Source: CAD feature listing. Evaluate the final solid. Frame: model axes, mm. Round coordinates to 2 decimals unless told otherwise and drop trailing zeros. Order: outer loops, then holes, each group sorted by start corner. A loop starts at its lowest first (then second) coordinate and runs counter-clockwise, first axis right, second up. Notation, with made-up numbers: (52.25, 40.5) - (83.25, 40.5) arc R17 ccw to (83.25, 60.5) - close; hole circle Ø3 at (75, 39). An arc over 180 degrees is marked (long way). Put each result on its own line as item: value. Start each with the question number.
1) Contact query for flat-ended pins moving along their axis: P1, Ø1.5, axis at x = 15.5, z = 45.5, coming from the +Y side; P2, Ø4, axis at y = -6.5, z = 30, coming from the -X side; P3, Ø4.5, axis at y = -6.5, z = 30, coming from the -X side; P4, Ø3.5, axis at x = -20, z = -50, coming from the -Y side. Output: stop coordinate, or through.
2) Section A-A on x = 20. Output: boundary loops of the cut face in (y, z), then the cut area to 3 significant figures.
3) Section C-C on x = 10.5. Output: boundary loops of the cut face in (y, z).
4) Section B-B on z = -50. Output: boundary loops of the cut face in (x, y).
5) Line query: probe 1 along Z at (x, y) = (20, -3.5); probe 2 along Z at (x, y) = (20.75, -6.5); probe 3 along Z at (x, y) = (-18.25, -6.5). Output: solid intervals per line, ascending. Write a range as [from, to].
```python
from build123d import *

# Parameters (mm, degrees)
F0_W     = 55
F0_H     = 115
F1_DEPTH = 13
F3_D     = 4.5
F3_DEPTH = 30
F3_TIP   = 1.3519363928
F5_D     = 5
F5_DEPTH = 20
F5_TIP   = 1.5021515476
F7_D     = 5
F7_DEPTH = 20
F7_TIP   = 1.5021515476
F8_R     = 5


with BuildPart() as f1:
    # F0 (on Front) → F1 (new body)
    with BuildSketch(Plane.XZ):
        Rectangle(F0_W, F0_H)
    extrude(amount=F1_DEPTH)

    # F3
    with Locations(Plane.XZ.offset(13)):
        with Locations((-20, 50), (20, 50), (20, -50), (-20, -50)):
            Hole(F3_D / 2, depth=F3_DEPTH)
            with Locations((0, 0, -(F3_DEPTH + F3_TIP / 2))):  # 118° drill point
                Cone(0, F3_D / 2, F3_TIP, mode=Mode.SUBTRACT)

    # F5
    with Locations(Plane.YZ.offset(27.5)):
        with Locations((-6.5, 30), (-6.5, -30)):
            Hole(F5_D / 2, depth=F5_DEPTH)
            with Locations((0, 0, -(F5_DEPTH + F5_TIP / 2))):  # 118° drill point
                Cone(0, F5_D / 2, F5_TIP, mode=Mode.SUBTRACT)

    # F7
    with Locations(Plane(origin=(-27.5, 0, 0), x_dir=(0, -1, 0), z_dir=(-1, 0, 0))):
        with Locations((6.5, 30), (6.5, -30)):
            Hole(F7_D / 2, depth=F7_DEPTH)
            with Locations((0, 0, -(F7_DEPTH + F7_TIP / 2))):  # 118° drill point
                Cone(0, F7_D / 2, F7_TIP, mode=Mode.SUBTRACT)

    # F8
    f8_edges = [f1.edges().sort_by_distance(p)[0] for p in [
        (27.5, -6.5, 57.5),
        (-27.5, -6.5, 57.5),
        (-27.5, -6.5, -57.5),
        (27.5, -6.5, -57.5),
    ]]
    fillet(f8_edges, radius=F8_R)


solid = f1.part
```
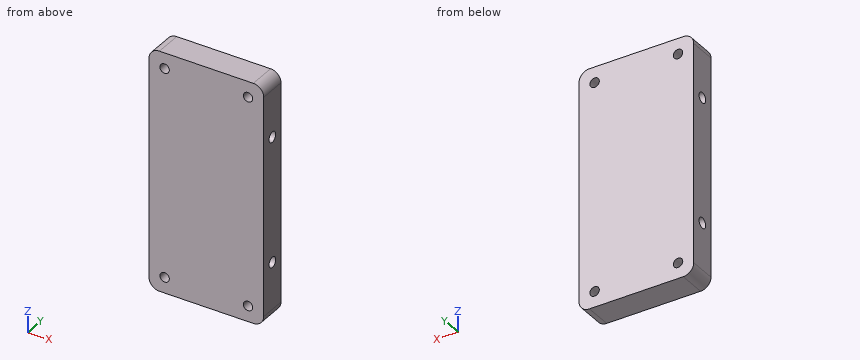
Answer sheet:
1. P1: y = 0
1. P2: x = -7.2
1. P3: x = -7.35
1. P4: through
2. outline: (-13, -57.5) - (0, -57.5) - (0, -52.25) - (-13, -52.25) - close; (-13, -47.75) - (0, -47.75) - (0, 47.75) - (-13, 47.75) - close; (-13, 52.25) - (0, 52.25) - (0, 57.5) - (-13, 57.5) - close; hole circle Ø5 at (-6.5, -30); hole circle Ø5 at (-6.5, 30)
2. area: 1,340 mm^2
3. outline: (-13, -57.5) - (0, -57.5) - (0, 57.5) - (-13, 57.5) - close; hole circle Ø5 at (-6.5, -30); hole circle Ø5 at (-6.5, 30)
4. outline: (-27.5, -13) - (-22.25, -13) - (-22.25, 0) - (-27.5, 0) - close; (-17.75, -13) - (17.75, -13) - (17.75, 0) - (-17.75, 0) - close; (22.25, -13) - (27.5, -13) - (27.5, 0) - (22.25, 0) - close
5. probe 1: [-57.5, -52.25], [-47.75, 47.75], [52.25, 57.5]
5. probe 2: [-57.5, -52.12], [-47.88, -32.5], [-27.5, 27.5], [32.5, 47.88], [52.12, 57.5]
5. probe 3: [-57.5, -51.41], [-48.59, -32.5], [-27.5, 27.5], [32.5, 48.59], [51.41, 57.5]
